Here's how the part is built. I have some questions about the finished solid (model axes, mm). A direction names the side the tool comes from. Round coordinates to 2 decimals unless told otherwise and drop trailing zeros. Loops run counter-clockwise (first coordinate to the right, second up) from the corner with the lowest first, then second, coordinate; pieces in that order, holes last. Notation, with made-up numbers: (58, 29) - (73, 29) arc R16 cw to (73, 45) - close; hole circle Ø2 at (-32.75, 84.5). An arc over 180 degrees is marked (long way). Answer as a JSON object with one key per item and string values. Group by question number.
1) I want a section at B-B, the plane y = -2. Please give me the cut outline in (x, z), then the cut area to 3 significant figures.
2) If we mould it in two halves opening along Y, with no side actions, what happens to faces 6 (the face through (0, 0, -4.762)), 7 (the face through (-6.95, -12.87, 0.07)), 8 (the face through (-5.74, -12.44, -0.07)), 9 (the face through (5.315, 9.223, -0.067))? For each: pulls with the +Y half, pulls with the -Y half, needs draft (parallel to the pull), parting line crosses it, or undercut.
3) I want a section at D-D, the plane x = 15.25. Please give me the cut outline in (y, z), then the cut area to 3 significant figures.
4) If I drill on line 1 along X through (y, z) = (0, -3.5); line 2 along Y through (x, z) = (1.5, 0.5); line 3 along Y through (x, z) = (-6.5, 3.25), over which ranges is the centre line in solid material (lowest first)? Write a range as [from, to].
5) Which directions (+Z, -Z, +X, -X, +Y, -Y) give clear straight access to the entire face, cutting with the end or side of a thin tool? Please do faces 1 (the face through (12.216, -25.607, 0.03)), 2 (the face through (12.5, -26.1, 2.159)), 3 (the face through (12.37, -23.93, 0.03)), 4 (the face through (12.5, -26.1, -2.159)), 5 (the face through (0, -13.906, 0)).
6) I want a section at C-C, the plane z = 3.5. Please give me the cut outline in (x, y).
7) Will these pins go through, and if not, where does the flat tip stop? P1, Ø10, axis at x = 11, y = -19, coming from the +Z side; P2, Ø4, axis at y = -13.5, z = 3, coming from the -X side; P3, Ø3, axis at x = 4, z = 2.5, coming from the -Y side.
8) I want a section at A-A, the plane z = 0.75. Please give me the cut outline in (x, y), then the cut area to 3 significant figures.
from build123d import *

# Parameters (mm, degrees)
SKETCH1_W                   = 15.875
SKETCH1_H                   = 27.813
BOSS_EXTRUDE1_DEPTH         = 4.7625
BOSS_EXTRUDE2_DEPTH         = 2.159
F_29_0_136_DIAMETER_HOLE1_D = 3.4544
FILLET1_R                   = 3.4544


with BuildPart() as part:
    # Sketch1 → Boss-Extrude1 (new, symmetric)
    with BuildSketch(Plane.XY):
        Rectangle(SKETCH1_W, SKETCH1_H)
    extrude(amount=BOSS_EXTRUDE1_DEPTH, both=True)

    # Sketch2 → Boss-Extrude2 (add, symmetric)
    with BuildSketch(Plane.XY):
        Polygon((7.9375, 1.2065), (16.926432647, -49.772270296), (16.376122074, -49.869304898), (7.9375, -0.655026961), align=None)
    extrude(amount=BOSS_EXTRUDE2_DEPTH, both=True)

    # #29 (0.136) Diameter Hole1 (through all)
    with Locations(Plane.XY.offset(4.7625)):
        with Locations((-4.9403, -10.9093), (4.9403, 10.9093)):
            Hole(F_29_0_136_DIAMETER_HOLE1_D / 2)

    # Fillet1
    fillet1_edges = [part.edges().sort_by_distance(p)[0] for p in [
        (-7.9375, -13.9065, 0),
        (7.9375, -13.9065, 0),
        (7.9375, 13.9065, 0),
        (-7.9375, 13.9065, 0),
    ]]
    fillet(fillet1_edges, radius=FILLET1_R)


solid = part.part
Outcome:
{
 "1": {"outline": "(-7.94, -4.76) - (7.94, -4.76) - (7.94, 4.76) - (-7.94, 4.76) - close; (8.17, -2.16) - (8.5, -2.16) - (8.5, 2.16) - (8.17, 2.16) - close", "area": "153 mm^2"},
 "2": {"face 6": "needs draft", "face 7": "pulls with the -Y half", "face 8": "undercut", "face 9": "undercut"},
 "3": {"outline": "(-43.3, -2.16) - (-40.26, -2.16) - (-40.26, 2.16) - (-43.3, 2.16) - close", "area": "13.1 mm^2"},
 "4": {"line 1": "[-7.94, 7.94]", "line 2": "[-13.91, 13.91]", "line 3": "[-13.26, -11.65], [-10.17, 13.26]"},
 "5": {"face 1": "+Z, -Z, -Y", "face 2": "+Z, +X, +Y, -Y", "face 3": "+Z, -Z, +X, +Y", "face 4": "-Z, +X, +Y, -Y", "face 5": "+Z, -Z, -X, -Y"},
 "6": {"outline": "(-7.94, -10.45) arc R3.45 ccw to (-4.48, -13.91) - (4.48, -13.91) arc R3.45 ccw to (7.94, -10.45) - (7.94, 10.45) arc R3.45 ccw to (4.48, 13.91) - (-4.48, 13.91) arc R3.45 ccw to (-7.94, 10.45) - close; hole circle Ø3.45 at (-4.94, -10.91); hole circle Ø3.45 at (4.94, 10.91)"},
 "7": {"P1": "z = 2.16", "P2": "x = -7.77", "P3": "y = -13.91"},
 "8": {"outline": "(-7.94, -10.45) arc R3.45 ccw to (-4.48, -13.91) - (4.48, -13.91) arc R3.45 ccw to (7.94, -10.45) - (7.94, -0.66) - (16.38, -49.87) - (16.93, -49.77) - (7.94, 1.21) - (7.94, 10.45) arc R3.45 ccw to (4.48, 13.91) - (-4.48, 13.91) arc R3.45 ccw to (-7.94, 10.45) - close; hole circle Ø3.45 at (-4.94, -10.91); hole circle Ø3.45 at (4.94, 10.91)", "area": "435 mm^2"}
}
